For this review, use the dimensioned drawing (mm, ordinates from the lowest corner) and the shaded views. Give positions to 0.01 mm unless a question says otherwise; leave off trailing zeros. Write each loop counter-clockwise with the first axis right and the second up, starting at its lowest first coordinate (ties: lowest second). Pieces come first, ordered by that corner, then holes. Notation, with made-up numbers: (-2.5, 79) -> (14.5, 79) arc R14 cw to (14.5, 98) -> close; hole circle Ø9 at (69.25, 52). An arc over 180 degrees is marked (long way). Write each question's results on one line, items separated by ' | '. Start each with the question number.
(1) Take a section at D-D (x = 2.75). State the section outline as (y, z) points, plus the area to 3 significant figures.
(2) Clearance check with a flat-ended pin moving along its axis: pin 1 (5.5 mm diameter, centred on x = 7, y = 16, fed in from +Z). State where the tip first meets the part, or that it passes through.
(3) Mouldability with a two-part tool opening along Y and no side actions: class the marked faces 1, 2 and 3 as released by +Y, released by -Y, zero draft, split by the parting line, or undercut.
(4) Take a section at A-A (z = 0.2). State the section outline as (x, y) points.
(5) Take a section at C-C (y = 3.5). State the section outline as (x, z) points.
(6) To check wall thickness, follow probe 1 along Y at (x, z) = (5.75, 0.3); probe 2 along Y at (x, z) = (7.5, 0.8); probe 3 along X at (y, z) = (20.5, 0.5). State the ranges of each line that lie inside material, in increasing order.
(7) Take a section at B-B (x = 7.25). State the section outline as (y, z) points.
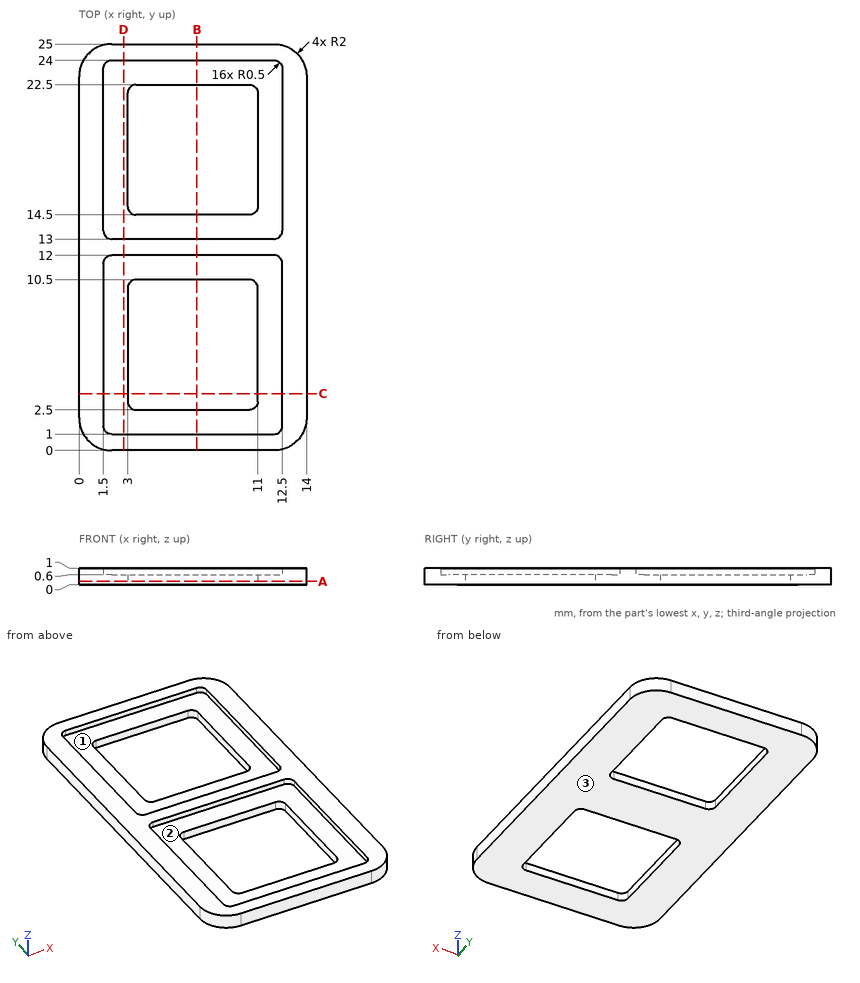
Report:
1) outline: (0, 0) -> (25, 0) -> (25, 1) -> (24, 1) -> (24, 0.6) -> (13, 0.6) -> (13, 1) -> (12, 1) -> (12, 0.6) -> (1, 0.6) -> (1, 1) -> (0, 1) -> close | area: 16.2 mm2
2) pin 1: z = 0.6
3) face 1: undercut | face 2: undercut | face 3: zero draft
4) outline: (0, 2) arc R2 ccw to (2, 0) -> (12, 0) arc R2 ccw to (14, 2) -> (14, 23) arc R2 ccw to (12, 25) -> (2, 25) arc R2 ccw to (0, 23) -> close; hole (3, 3) arc R0.5 ccw to (3.5, 2.5) -> (10.5, 2.5) arc R0.5 ccw to (11, 3) -> (11, 10) arc R0.5 ccw to (10.5, 10.5) -> (3.5, 10.5) arc R0.5 ccw to (3, 10) -> close; hole (3, 15) arc R0.5 ccw to (3.5, 14.5) -> (10.5, 14.5) arc R0.5 ccw to (11, 15) -> (11, 22) arc R0.5 ccw to (10.5, 22.5) -> (3.5, 22.5) arc R0.5 ccw to (3, 22) -> close
5) outline: (0, 0) -> (3, 0) -> (3, 0.6) -> (1.5, 0.6) -> (1.5, 1) -> (0, 1) -> close; (11, 0) -> (14, 0) -> (14, 1) -> (12.5, 1) -> (12.5, 0.6) -> (11, 0.6) -> close
6) probe 1: 0 to 2.5, 10.5 to 14.5, 22.5 to 25 | probe 2: 0 to 1, 12 to 13, 24 to 25 | probe 3: 0 to 3, 11 to 14
7) outline: (0, 0) -> (2.5, 0) -> (2.5, 0.6) -> (1, 0.6) -> (1, 1) -> (0, 1) -> close; (10.5, 0) -> (14.5, 0) -> (14.5, 0.6) -> (13, 0.6) -> (13, 1) -> (12, 1) -> (12, 0.6) -> (10.5, 0.6) -> close; (22.5, 0) -> (25, 0) -> (25, 1) -> (24, 1) -> (24, 0.6) -> (22.5, 0.6) -> close
